Source: three-view drawing plus pictorial views. Frame: mm from the lowest corner of the part. Give positions to 0.01 mm unless a question says otherwise; leave off trailing zeros. Loops run counter-clockwise (first coordinate to the right, second up) from the corner with the lowest first, then second, coordinate; pieces in that order, holes last.
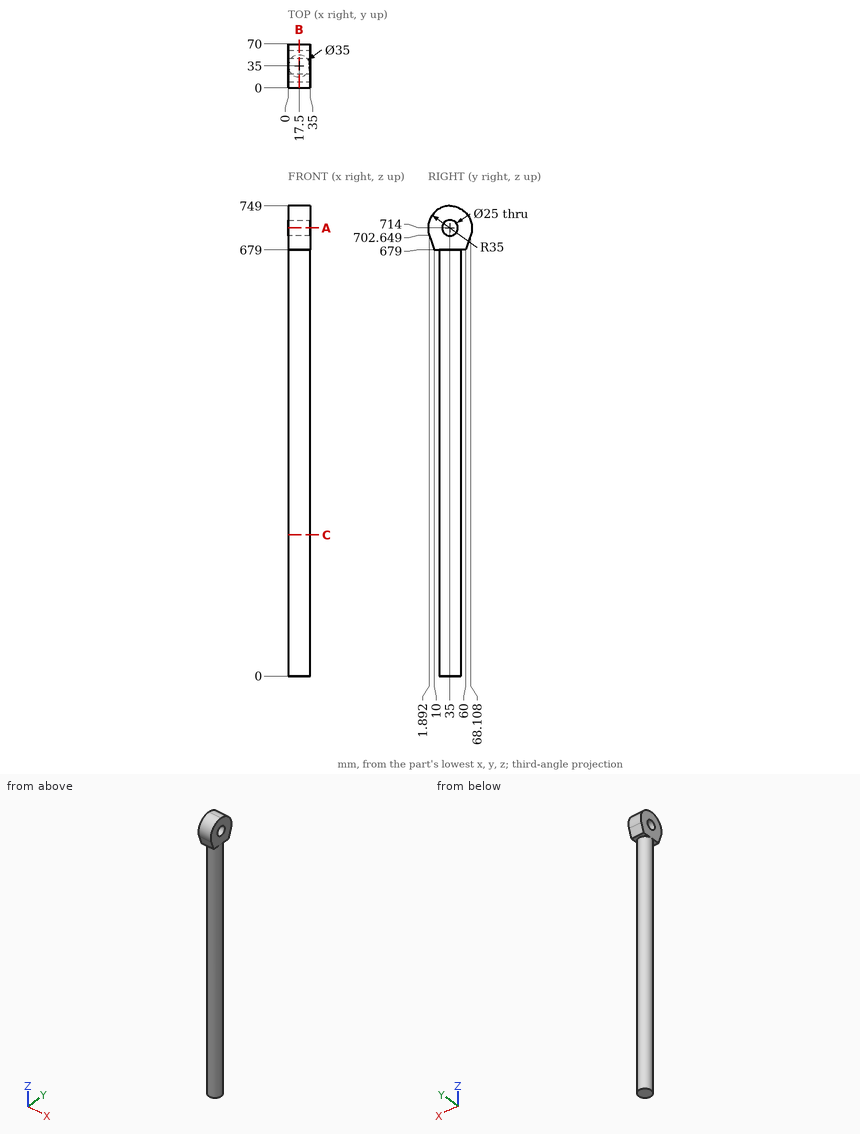
(1) Cut plane B-B (x = 17.5). Return the cut outline in (y, z).
Values follow:
outline: (1.89, 702.65) - (10, 679) - (17.5, 679) - (17.5, 0) - (52.5, 0) - (52.5, 679) - (60, 679) - (68.11, 702.65) arc R35 ccw (long way) to start; hole circle Ø25 at (35, 714)
(2) Cut plane C-C (z = 225). Return the cut outline in (x, y), and give its area (3 significant figures).
Values follow:
outline: circle Ø35 at (17.5, 35)
area: 962 mm2
(3) Ray query, probe 1 along Z at (x, y) = (32.5, 36) (1 decimal); probe 2 along Y at (x, z) = (21.5, 714); probe 3 along X at (y, z) = (37, 418.5) (1 decimal). Return the intervals inside material, ascending.
Values follow:
probe 1: z = 0 to 701.5, 726.5 to 749
probe 2: y = 0 to 22.5, 47.5 to 70
probe 3: x = 0.1 to 34.9
(4) Pin query (flat end, axial travel): pin 1 Ø6 at (x, y) = (26, 10.5) entering from +Z; pin 2 Ø10 at (x, y) = (26.5, 23.5) entering from +Z; pin 3 Ø3 at (x, z) = (27.5, 367.5) entering from -Y. Return the tip coordinate at first contact, or that it passes through.
Values follow:
pin 1: stops at z = 741.62
pin 2: stops at z = 748.39
pin 3: stops at y = 19.7
(5) Cut plane A-A (z = 714). Return the cut outline in (x, y), and give its area (4 significant figures).
Values follow:
outline: (0, 0) - (35, 0) - (35, 22.5) - (0, 22.5) - close; (0, 47.5) - (35, 47.5) - (35, 70) - (0, 70) - close
area: 1,575 mm2
